Can you work these out from the model? Positions are in its coordinate system, mm. A direction names the side the tool comes from. Coordinates: 2 decimals unless noted, no trailing zeros. Order: outer loops, then holes, each group sorted by start corner. A loop starts at its lowest first (then second) coordinate and runs counter-clockwise, first axis right, second up. Notation, with made-up numbers: M 47,2 L 52,2 A21 ccw 52,39 Z; hole C 2.5,62.25 d6. An arc over 180 degrees is marked long. Answer as CSV lines item,"result". Start each with the question number.
1. If we section it at A-A (z = -16): List the corners of the cut face in (x, y) for me.
2. On a 3-axis mill with a long thin cutter (end or side, diameter ignored), from which of +Z, -Z, +X, -X, +Y, -Y can I reach the whole of each face in a straight line? I mean faces 1 (the face through (48, -1, -19.05)), 2 (the face through (-1, -2.972, 0)). Say none if no direction works.
3. If we section it at B-B (y = -0.55): Give the number of separate pieces and of enclosed holes in the cut face, plus the area to 3 significant figures.
4. I need wall thicknesses on line 1 along X through (y, z) = (-1.85, -28) (3 decimals); line 2 along Z through (x, y) = (-0.5, -1); line 3 along X through (y, z) = (-1.6, 16.5). Which ranges of each line are inside material? Lowest first, please. Write a range as from..to.
5. If we mould it in two halves opening along Z, with no side actions, what happens to faces 3 (the face through (-1, -1, -31.75)), 4 (the face through (49.53, -1, -16)), 5 (the face through (0, -1, -30.48)), 6 (the face through (50.8, -1, 0))? For each: released by +Z, released by -Z, zero draft, split by the parting line, or undercut.
```python
from build123d import *

# Parameters (mm, degrees)
F0_W     = 101.6
F0_H     = 63.5
F0_W_2   = 6.35
F0_H_2   = 2.9718
F0_W_3   = 2.9718
F0_H_3   = 6.35
F1_DEPTH = 2.9718


with BuildPart() as f1:
    # F0 (on Front) → F1 (new body)
    with BuildSketch(Plane.XZ):
        Rectangle(F0_W, F0_H)
        with Locations((-34.925, -28.9941)):
            Rectangle(F0_W_2, F0_H_2, mode=Mode.SUBTRACT)
        with Locations((0, -28.9941)):
            Rectangle(F0_W_2, F0_H_2, mode=Mode.SUBTRACT)
        with Locations((-48.0441, -15.875)):
            Rectangle(F0_W_3, F0_H_3, mode=Mode.SUBTRACT)
        with Locations((34.925, -28.9941)):
            Rectangle(F0_W_2, F0_H_2, mode=Mode.SUBTRACT)
        with Locations((48.0441, -15.875)):
            Rectangle(F0_W_3, F0_H_3, mode=Mode.SUBTRACT)
        with Locations((-48.0441, 15.875)):
            Rectangle(F0_W_3, F0_H_3, mode=Mode.SUBTRACT)
        with Locations((0, 28.9941)):
            Rectangle(F0_W_2, F0_H_2, mode=Mode.SUBTRACT)
        with Locations((48.0441, 15.875)):
            Rectangle(F0_W_3, F0_H_3, mode=Mode.SUBTRACT)
    extrude(amount=F1_DEPTH)


solid = f1.part
```
Solved:
1,outline,"M -50.8,-2.97 L -49.53,-2.97 L -49.53,0 L -50.8,0 Z; M -46.56,-2.97 L 46.56,-2.97 L 46.56,0 L -46.56,0 Z; M 49.53,-2.97 L 50.8,-2.97 L 50.8,0 L 49.53,0 Z"
2,face 1,"+Y, -Y"
2,face 2,"+Z, -Z, +X, -X, -Y"
3,separate pieces,"1"
3,enclosed holes,"8"
3,area,"6,300 mm²"
4,line 1,"-50.8..-38.1, -31.75..-3.175, 3.175..31.75, 38.1..50.8"
4,line 2,"-31.75..-30.48, -27.51..27.51, 30.48..31.75"
4,line 3,"-50.8..-49.53, -46.56..46.56, 49.53..50.8"
5,face 3,"released by -Z"
5,face 4,"undercut"
5,face 5,"undercut"
5,face 6,"zero draft"
